Geometry: final body of the model. Coordinates: model frame, mm. Face numbers are marked on the shaded views. A direction names the side the tool comes from. Give positions to 0.01 mm unless a question says otherwise; leave off trailing zeros. Write each loop counter-clockwise with the first axis right and the second up, starting at its lowest first coordinate (ties: lowest second). Pieces come first, ordered by that corner, then holes. Notation, with made-up numbers: (-31.75, 87.5) -> (14.25, 87.5) arc R18 ccw to (14.25, 110.5) -> close; hole circle Ø1 at (-1, 55.25). An arc over 180 degrees is marked (long way). Use CSV: the item, a comma, the result in double quotes. Start each with the question number.
1) Set-up query: the marked faces 1, 2 and 3. Return all of +Z, -Z, +X, -X, +Y, -Y with unobstructed straight access to the full face (end or side cutting, diameter ignored); none if empty.
2) Contact query for flat-ended pins moving along their axis: P1, Ø6, axis at y = 0, z = 14.5, coming from the -X side; P2, Ø1, axis at y = -3, z = 15, coming from the +X side; P3, Ø4, axis at y = -4.5, z = 13.5, coming from the -X side; P4, Ø5, axis at x = 30.5, z = 7, coming from the -Y side. Output: stop coordinate, or through.
3) Draft query along Z for the marked faces 4, 5, 6 and 7. Return one class per face: pulls with the +Z half, pulls with the -Z half, needs draft (parallel to the pull), parting line crosses it, or undercut.
4) Material intervals for line 1 (Z direction, x = 57.5, y = -2.25); line 2 (X direction, y = 1.25, z = 12.5); line 3 (Y direction, x = 36, z = 5.5), sorted ascending. Write a range as [from, to].
5) Section A-A (z = 10). Output: boundary loops of the cut face in (x, y), plus the area to 3 significant figures.
6) Section B-B (z = 2.75). Output: boundary loops of the cut face in (x, y), plus the area to 3 significant figures.
```python
from build123d import *
from OCP.BRepFilletAPI import BRepFilletAPI_MakeChamfer

# Parameters (mm, degrees)
BOSS_EXTRUDE1_DEPTH = 20
CUT_EXTRUDE1_REACH  = 67.044
FILLET1_R           = 2
CHAMFER1_SIZE       = 2
CHAMFER1_SIZE2      = 1.154700538
CHAMFER2_SIZE       = 2
CHAMFER2_SIZE2      = 1.154700538
FILLET2_R           = 1
FILLET3_R           = 0.5


with BuildPart() as part:
    # Sketch1 → Boss-Extrude1 (new body)
    with BuildSketch(Plane.XY):
        with BuildLine():
            Line((0, 0), (8, 0))
            Line((8, 0), (8, -3))
            Line((8, -3), (40.754109963, -3))
            ThreePointArc((40.754109963, -3), (51.941790363, -9), (60, 0.809661064))
            Line((60, 0.809661064), (60, 6))
            Line((60, 6), (0, 6))
            Line((0, 6), (0, 0))
        make_face()
    extrude(amount=BOSS_EXTRUDE1_DEPTH)

    # Sketch2 → Cut-Extrude1 (cut, up to next)
    with BuildSketch(Plane(origin=(0, 6, 0), x_dir=(1, 0, 0), z_dir=(0, 1, 0)), mode=Mode.PRIVATE) as cut_extrude1_sk1:
        with BuildLine():
            Line((25.5, -5.85), (30.5, -5.85))
            ThreePointArc((30.5, -5.85), (34.65, -10), (30.5, -14.15))
            Line((30.5, -14.15), (25.5, -14.15))
            ThreePointArc((25.5, -14.15), (21.35, -10), (25.5, -5.85))
        make_face()
    cut_extrude1_tool1 = extrude(cut_extrude1_sk1.sketch, amount=-CUT_EXTRUDE1_REACH, mode=Mode.PRIVATE) & part.part
    add(cut_extrude1_tool1.solids().sort_by_distance((28, 6, 10))[0], mode=Mode.SUBTRACT)

    # Fillet1
    fillet1_edges = [part.edges().sort_by_distance(p)[0] for p in [
        (0, 3, 0),
        (8, -1.5, 20),
        (40.754109963, -3, 10),
        (8, -3, 10),
        (0, 0, 10),
        (24.377054981, -3, 20),
        (51.941790363, -9, 20),
        (60, 3.404830532, 20),
        (0, 3, 20),
        (60, 3.404830532, 0),
        (51.941790363, -9, 0),
        (24.377054981, -3, 0),
        (4, 0, 20),
        (8, -1.5, 0),
        (4, 0, 0),
    ]]
    fillet(fillet1_edges, radius=FILLET1_R)

    # Chamfer1: one chamfer whose edges measure the first distance from different faces: ONE call of the kernel's chamfer builder (chamfer() names one face for all edges)
    chamfer1_edges_1 = [part.edges().sort_by_distance(p)[0] for p in [
        (30, 6, 0),
    ]]
    chamfer1_side_1 = [part.faces().sort_by_distance(p)[0] for p in [
        (34.587898507, 1.608386823, 0),
    ]]
    chamfer1_edges_2 = [part.edges().sort_by_distance(p)[0] for p in [
        (30, 6, 20),
    ]]
    chamfer1_side_2 = [part.faces().sort_by_distance(p)[0] for p in [
        (34.587898507, 1.608386823, 20),
    ]]
    chamfer1_edges_3 = [part.edges().sort_by_distance(p)[0] for p in [
        (60, 6, 10),
    ]]
    chamfer1_side_3 = [part.faces().sort_by_distance(p)[0] for p in [
        (60, 3.404830532, 10),
    ]]
    chamfer1_edges_4 = [part.edges().sort_by_distance(p)[0] for p in [
        (0, 6, 10),
    ]]
    chamfer1_side_4 = [part.faces().sort_by_distance(p)[0] for p in [
        (0, 4, 10),
    ]]
    chamfer1_edges_5 = [part.edges().sort_by_distance(p)[0] for p in [
        (0.585786438, 6, 19.414213562),
    ]]
    chamfer1_side_5 = [part.faces().sort_by_distance(p)[0] for p in [
        (0.585786438, 4, 19.414213562),
    ]]
    chamfer1_edges_6 = [part.edges().sort_by_distance(p)[0] for p in [
        (0.585786438, 6, 0.585786438),
    ]]
    chamfer1_side_6 = [part.faces().sort_by_distance(p)[0] for p in [
        (0.585786438, 4, 0.585786438),
    ]]
    chamfer1_edges_7 = [part.edges().sort_by_distance(p)[0] for p in [
        (59.414213562, 6, 19.414213562),
    ]]
    chamfer1_side_7 = [part.faces().sort_by_distance(p)[0] for p in [
        (59.414213562, 3.404830532, 19.414213562),
    ]]
    chamfer1_edges_8 = [part.edges().sort_by_distance(p)[0] for p in [
        (59.414213562, 6, 0.585786438),
    ]]
    chamfer1_side_8 = [part.faces().sort_by_distance(p)[0] for p in [
        (59.414213562, 3.404830532, 0.585786438),
    ]]
    chamfer1 = BRepFilletAPI_MakeChamfer(part.part.solid().wrapped)
    for e in chamfer1_edges_1:
        chamfer1.Add(CHAMFER1_SIZE, CHAMFER1_SIZE2, e.wrapped, chamfer1_side_1[0].wrapped)  # the first distance lies on this face
    for e in chamfer1_edges_2:
        chamfer1.Add(CHAMFER1_SIZE, CHAMFER1_SIZE2, e.wrapped, chamfer1_side_2[0].wrapped)  # the first distance lies on this face
    for e in chamfer1_edges_3:
        chamfer1.Add(CHAMFER1_SIZE, CHAMFER1_SIZE2, e.wrapped, chamfer1_side_3[0].wrapped)  # the first distance lies on this face
    for e in chamfer1_edges_4:
        chamfer1.Add(CHAMFER1_SIZE, CHAMFER1_SIZE2, e.wrapped, chamfer1_side_4[0].wrapped)  # the first distance lies on this face
    for e in chamfer1_edges_5:
        chamfer1.Add(CHAMFER1_SIZE, CHAMFER1_SIZE2, e.wrapped, chamfer1_side_5[0].wrapped)  # the first distance lies on this face
    for e in chamfer1_edges_6:
        chamfer1.Add(CHAMFER1_SIZE, CHAMFER1_SIZE2, e.wrapped, chamfer1_side_6[0].wrapped)  # the first distance lies on this face
    for e in chamfer1_edges_7:
        chamfer1.Add(CHAMFER1_SIZE, CHAMFER1_SIZE2, e.wrapped, chamfer1_side_7[0].wrapped)  # the first distance lies on this face
    for e in chamfer1_edges_8:
        chamfer1.Add(CHAMFER1_SIZE, CHAMFER1_SIZE2, e.wrapped, chamfer1_side_8[0].wrapped)  # the first distance lies on this face
    add(Compound.cast(chamfer1.Shape()), mode=Mode.REPLACE)

    # Chamfer2: one chamfer whose edges measure the first distance from different faces: ONE call of the kernel's chamfer builder (chamfer() names one face for all edges)
    chamfer2_edges_1 = [part.edges().sort_by_distance(p)[0] for p in [
        (21.35, 6, 10),
    ]]
    chamfer2_side_1 = [part.faces().sort_by_distance(p)[0] for p in [
        (21.35, 1.5, 10),
    ]]
    chamfer2_edges_2 = [part.edges().sort_by_distance(p)[0] for p in [
        (28, 6, 14.15),
    ]]
    chamfer2_side_2 = [part.faces().sort_by_distance(p)[0] for p in [
        (28, 1.5, 14.15),
    ]]
    chamfer2_edges_3 = [part.edges().sort_by_distance(p)[0] for p in [
        (34.65, 6, 10),
    ]]
    chamfer2_side_3 = [part.faces().sort_by_distance(p)[0] for p in [
        (34.65, 1.5, 10),
    ]]
    chamfer2_edges_4 = [part.edges().sort_by_distance(p)[0] for p in [
        (28, 6, 5.85),
    ]]
    chamfer2_side_4 = [part.faces().sort_by_distance(p)[0] for p in [
        (28, 1.5, 5.85),
    ]]
    chamfer2 = BRepFilletAPI_MakeChamfer(part.part.solid().wrapped)
    for e in chamfer2_edges_1:
        chamfer2.Add(CHAMFER2_SIZE, CHAMFER2_SIZE2, e.wrapped, chamfer2_side_1[0].wrapped)  # the first distance lies on this face
    for e in chamfer2_edges_2:
        chamfer2.Add(CHAMFER2_SIZE, CHAMFER2_SIZE2, e.wrapped, chamfer2_side_2[0].wrapped)  # the first distance lies on this face
    for e in chamfer2_edges_3:
        chamfer2.Add(CHAMFER2_SIZE, CHAMFER2_SIZE2, e.wrapped, chamfer2_side_3[0].wrapped)  # the first distance lies on this face
    for e in chamfer2_edges_4:
        chamfer2.Add(CHAMFER2_SIZE, CHAMFER2_SIZE2, e.wrapped, chamfer2_side_4[0].wrapped)  # the first distance lies on this face
    add(Compound.cast(chamfer2.Shape()), mode=Mode.REPLACE)

    # Fillet2
    fillet2_edges = [part.edges().sort_by_distance(p)[0] for p in [
        (28, -3, 14.15),
        (21.35, -3, 10),
        (28, -3, 5.85),
        (34.65, -3, 10),
    ]]
    fillet(fillet2_edges, radius=FILLET2_R)

    # Fillet3
    fillet3_edges = [part.edges().sort_by_distance(p)[0] for p in [
        (8, 0, 10),
        (8.707902185, 0.707902185, 19.526592034),
        (8.707902185, 0.707902185, 0.473407966),
    ]]
    fillet(fillet3_edges, radius=FILLET3_R)


solid = part.part
```
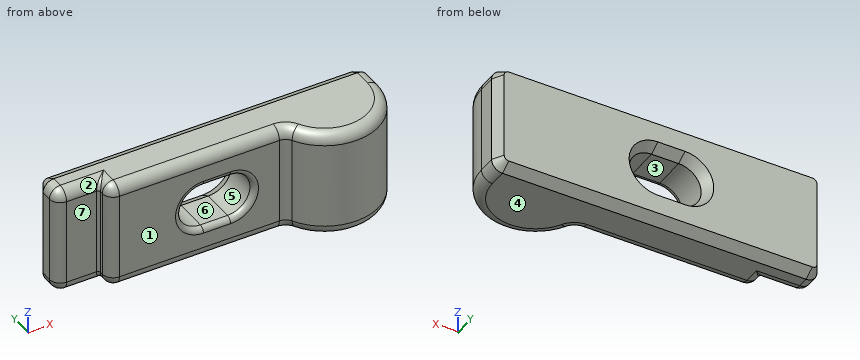
Answers follow:
1,face 1,"+Z, -Z, -X, -Y"
1,face 2,"+Z, -X, -Y"
1,face 3,"+Y, -Y"
2,P1,"stops at x = 0"
2,P2,"stops at x = 59.44"
2,P3,"stops at x = 8.68"
2,P4,"stops at y = -3"
3,face 4,"pulls with the -Z half"
3,face 5,"undercut"
3,face 6,"undercut"
3,face 7,"needs draft"
4,line 1,"z = [0, 20]"
4,line 2,"x = [0.15, 22.19], [33.81, 60]"
4,line 3,"y = [-3, 6]"
5,outline,"(0, 2) arc R2 ccw to (2, 0) -> (7.5, 0) arc R0.5 cw to (8, -0.5) -> (8, -1) arc R2 ccw to (10, -3) -> (20.35, -3) arc R1 ccw to (21.35, -2) -> (21.35, 4) -> (20.2, 6) -> (1.15, 6) -> (0, 4) -> close; (34.65, -2) arc R1 ccw to (35.65, -3) -> (39.5, -3) arc R2 cw to (41.25, -4.03) arc R10 ccw to (60, 0.81) -> (60, 4) -> (58.85, 6) -> (35.8, 6) -> (34.65, 4) -> close"
5,area,"472 mm^2"
6,outline,"(0, 2) arc R2 ccw to (2, 0) -> (7.5, 0) arc R0.5 cw to (8, -0.5) -> (8, -1) arc R2 ccw to (10, -3) -> (39.5, -3) arc R2 cw to (41.25, -4.03) arc R10 ccw to (60, 0.81) -> (60, 4) -> (58.85, 6) -> (1.15, 6) -> (0, 4) -> close"
6,area,"594 mm^2"
